Here's how the part is built. I have some questions about the finished solid (model axes, mm). A direction names the side the tool comes from. Coordinates: 2 decimals unless noted, no trailing zeros. Use one line per item in the form item = value. Start each with the question number.
from build123d import *

# Parameters (mm, degrees)
SKETCH1_R           = 4
SKETCH1_W           = 4
SKETCH1_H           = 4
BOSS_EXTRUDE1_DEPTH = 500


with BuildPart() as part:
    # Sketch1 → Boss-Extrude1 (new body)
    with BuildSketch(Plane.XY):
        with BuildLine():
            Line((-15, -4), (-15, -13))
            ThreePointArc((-15, -13), (-14.414213562, -14.414213562), (-13, -15))
            Line((-13, -15), (-4, -15))
            Line((-4, -15), (-4, -12.75))
            Line((-4, -12.75), (-7.5, -12.75))
            ThreePointArc((-7.5, -12.75), (-8.207106781, -12.457106781), (-8.5, -11.75))
            Line((-8.5, -11.75), (-8.5, -10.681980515))
            ThreePointArc((-8.5, -10.681980515), (-8.423879533, -10.299297083), (-8.207106781, -9.974873734))
            Line((-8.207106781, -9.974873734), (-4.525126266, -6.292893219))
            ThreePointArc((-4.525126266, -6.292893219), (-4.200702917, -6.076120467), (-3.818019485, -6))
            Line((-3.818019485, -6), (3.818019485, -6))
            ThreePointArc((3.818019485, -6), (4.200702917, -6.076120467), (4.525126266, -6.292893219))
            Line((4.525126266, -6.292893219), (8.207106781, -9.974873734))
            ThreePointArc((8.207106781, -9.974873734), (8.423879533, -10.299297083), (8.5, -10.681980515))
            Line((8.5, -10.681980515), (8.5, -11.75))
            ThreePointArc((8.5, -11.75), (8.207106781, -12.457106781), (7.5, -12.75))
            Line((7.5, -12.75), (4, -12.75))
            Line((4, -12.75), (4, -15))
            Line((4, -15), (13, -15))
            ThreePointArc((13, -15), (14.414213562, -14.414213562), (15, -13))
            Line((15, -13), (15, -4))
            Line((15, -4), (12.75, -4))
            Line((12.75, -4), (12.75, -8.5))
            Line((12.75, -8.5), (10.267766953, -8.5))
            Line((10.267766953, -8.5), (6.292893219, -4.525126266))
            ThreePointArc((6.292893219, -4.525126266), (6.076120467, -4.200702917), (6, -3.818019485))
            Line((6, -3.818019485), (6, 3.818019485))
            ThreePointArc((6, 3.818019485), (6.076120467, 4.200702917), (6.292893219, 4.525126266))
            Line((6.292893219, 4.525126266), (9.974873734, 8.207106781))
            ThreePointArc((9.974873734, 8.207106781), (10.299297083, 8.423879533), (10.681980515, 8.5))
            Line((10.681980515, 8.5), (11.75, 8.5))
            ThreePointArc((11.75, 8.5), (12.457106781, 8.207106781), (12.75, 7.5))
            Line((12.75, 7.5), (12.75, 4))
            Line((12.75, 4), (15, 4))
            Line((15, 4), (15, 13))
            ThreePointArc((15, 13), (14.414213562, 14.414213562), (13, 15))
            Line((13, 15), (4, 15))
            Line((4, 15), (4, 12.75))
            Line((4, 12.75), (7.5, 12.75))
            ThreePointArc((7.5, 12.75), (8.207106781, 12.457106781), (8.5, 11.75))
            Line((8.5, 11.75), (8.5, 10.681980515))
            ThreePointArc((8.5, 10.681980515), (8.423879533, 10.299297083), (8.207106781, 9.974873734))
            Line((8.207106781, 9.974873734), (4.525126266, 6.292893219))
            ThreePointArc((4.525126266, 6.292893219), (4.200702917, 6.076120467), (3.818019485, 6))
            Line((3.818019485, 6), (-3.818019485, 6))
            ThreePointArc((-3.818019485, 6), (-4.200702917, 6.076120467), (-4.525126266, 6.292893219))
            Line((-4.525126266, 6.292893219), (-8.207106781, 9.974873734))
            ThreePointArc((-8.207106781, 9.974873734), (-8.423879533, 10.299297083), (-8.5, 10.681980515))
            Line((-8.5, 10.681980515), (-8.5, 11.75))
            ThreePointArc((-8.5, 11.75), (-8.207106781, 12.457106781), (-7.5, 12.75))
            Line((-7.5, 12.75), (-4, 12.75))
            Line((-4, 12.75), (-4, 15))
            Line((-4, 15), (-13, 15))
            ThreePointArc((-13, 15), (-14.414213562, 14.414213562), (-15, 13))
            Line((-15, 13), (-15, 4))
            Line((-15, 4), (-12.75, 4))
            Line((-12.75, 4), (-12.75, 7.5))
            ThreePointArc((-12.75, 7.5), (-12.457106781, 8.207106781), (-11.75, 8.5))
            Line((-11.75, 8.5), (-10.681980515, 8.5))
            ThreePointArc((-10.681980515, 8.5), (-10.299297083, 8.423879533), (-9.974873734, 8.207106781))
            Line((-9.974873734, 8.207106781), (-6.292893219, 4.525126266))
            ThreePointArc((-6.292893219, 4.525126266), (-6.076120467, 4.200702917), (-6, 3.818019485))
            Line((-6, 3.818019485), (-6, -3.818019485))
            ThreePointArc((-6, -3.818019485), (-6.076120467, -4.200702917), (-6.292893219, -4.525126266))
            Line((-6.292893219, -4.525126266), (-9.974873734, -8.207106781))
            ThreePointArc((-9.974873734, -8.207106781), (-10.299297083, -8.423879533), (-10.681980515, -8.5))
            Line((-10.681980515, -8.5), (-11.75, -8.5))
            ThreePointArc((-11.75, -8.5), (-12.457106781, -8.207106781), (-12.75, -7.5))
            Line((-12.75, -7.5), (-12.75, -4))
            Line((-12.75, -4), (-15, -4))
        make_face()
        Circle(SKETCH1_R, mode=Mode.SUBTRACT)
        with BuildLine():
            Line((9.75, -10.75), (9.75, -12.75))
            ThreePointArc((9.75, -12.75), (10.042893219, -13.457106781), (10.75, -13.75))
            Line((10.75, -13.75), (12.75, -13.75))
            ThreePointArc((12.75, -13.75), (13.457106781, -13.457106781), (13.75, -12.75))
            Line((13.75, -12.75), (13.75, -10.75))
            ThreePointArc((13.75, -10.75), (13.457106781, -10.042893219), (12.75, -9.75))
            Line((12.75, -9.75), (10.75, -9.75))
            ThreePointArc((10.75, -9.75), (10.042893219, -10.042893219), (9.75, -10.75))
        make_face(mode=Mode.SUBTRACT)
        with Locations((11.75, 11.75)):
            Rectangle(SKETCH1_W, SKETCH1_H, mode=Mode.SUBTRACT)
        with BuildLine():
            Line((-10.75, 13.75), (-12.75, 13.75))
            ThreePointArc((-12.75, 13.75), (-13.457106781, 13.457106781), (-13.75, 12.75))
            Line((-13.75, 12.75), (-13.75, 10.75))
            ThreePointArc((-13.75, 10.75), (-13.457106781, 10.042893219), (-12.75, 9.75))
            Line((-12.75, 9.75), (-10.75, 9.75))
            ThreePointArc((-10.75, 9.75), (-10.042893219, 10.042893219), (-9.75, 10.75))
            Line((-9.75, 10.75), (-9.75, 12.75))
            ThreePointArc((-9.75, 12.75), (-10.042893219, 13.457106781), (-10.75, 13.75))
        make_face(mode=Mode.SUBTRACT)
        with BuildLine():
            Line((-12.75, -13.75), (-10.75, -13.75))
            ThreePointArc((-10.75, -13.75), (-10.042893219, -13.457106781), (-9.75, -12.75))
            Line((-9.75, -12.75), (-9.75, -10.75))
            ThreePointArc((-9.75, -10.75), (-10.042893219, -10.042893219), (-10.75, -9.75))
            Line((-10.75, -9.75), (-12.75, -9.75))
            ThreePointArc((-12.75, -9.75), (-13.457106781, -10.042893219), (-13.75, -10.75))
            Line((-13.75, -10.75), (-13.75, -12.75))
            ThreePointArc((-13.75, -12.75), (-13.457106781, -13.457106781), (-12.75, -13.75))
        make_face(mode=Mode.SUBTRACT)
    extrude(amount=BOSS_EXTRUDE1_DEPTH)


solid = part.part
1) Which directions (+Z, -Z, +X, -X, +Y, -Y) give clear straight access to the entire face, cutting with the end or side of a thin tool? Please do faces 5 (the flat face through (0, 6, 246)), 6 (the flat face through (0, -6, 246)), 7 (the flat face through (-6, 0, 246)), 8 (the flat face through (8, -15, 246)), 9 (the flat face through (15, -9, 246)).
2) For pin 1 (1.5 mm diameter, centred on y = 0.5, z = 194.5, fed in from +X), with a flat end and sliding along its axis, tell me the tip position at first contact or that it passes through.
3) I need wall thicknesses on probe 1 along X at (y, z) = (-13, 288.5); probe 2 along Y at (x, z) = (-12.5, 61.5); probe 3 along X at (y, z) = (-1, 467). Which ranges of each line are inside material? Lowest first, please. Write a range as [from, to].
4) If we mould it in two halves opening along Y, with no side actions, what happens to faces 1 (the flat face through (15, 8, 246)), 2 (the flat face through (6, 0, 246)), 3 (the cylindrical face through (-0.867, -3.905, 246.5)), 4 (the flat face through (9, 15, 246))? For each: pulls with the +Y half, pulls with the -Y half, needs draft (parallel to the pull), parting line crosses it, or undercut.
5) Suppose I cut it at A-A, the plane z = 363.5. Give the number of separate pieces and of enclosed holes in the cut face, then the cut area to 3 significant figures.
From the geometry:
q1.face_5 = +Z, -Z, +Y
q1.face_6 = +Z, -Z, -Y
q1.face_7 = +Z, -Z, -X
q1.face_8 = +Z, -Z, +X, -X, -Y
q1.face_9 = +Z, -Z, +X, +Y, -Y
q2.pin_1 = 6
q3.probe_1 = [-15, -13.72], [-9.78, -4], [4, 9.78], [13.72, 15]
q3.probe_2 = [-15, -13.75], [-9.75, -8.16], [8.16, 9.75], [13.75, 15]
q3.probe_3 = [-6, -3.87], [3.87, 6]
q4.face_1 = needs draft
q4.face_2 = undercut
q4.face_3 = undercut
q4.face_4 = pulls with the +Y half
q5.separate_pieces = 1
q5.enclosed_holes = 5
q5.area = 329 mm2
